from build123d import *

# Parameters (mm, degrees)
F1_DEPTH = 15
F2_R     = 7.63
F3_DEPTH = 15.001


with BuildPart() as f1:
    # F0 (on Front) → F1 (new body)
    with BuildSketch(Plane.XZ):
        Polygon((-7.649891, 13.25), (-15.299782, 0), (-7.649891, -13.25), (7.649891, -13.25), (15.299782, 0), (7.649891, 13.25), align=None)
    extrude(amount=F1_DEPTH)

    # F2 (on face) → F3 (cut, through all)
    with BuildSketch(Plane.XZ.offset(15)):
        Circle(F2_R)
    extrude(amount=-F3_DEPTH, mode=Mode.SUBTRACT)


solid = f1.part
Could you check a few things on this model? Use its own coordinates, in mm. Round coordinates to 2 decimals unless told otherwise and drop trailing zeros. Write each loop counter-clockwise with the first axis right and the second up, starting at its lowest first coordinate (ties: lowest second). Pieces come first, ordered by that corner, then holes. Notation, with made-up numbers: (-25.75, 23) -> (-13.75, 23) arc R5 cw to (-13.75, 30) -> close; hole circle Ø7 at (-13, 48). An arc over 180 degrees is marked (long way). Use a Markdown table: item, result.
1. If we section it at D-D (z = -8.25): List the corners of the cut face in (x, y) for me.
Answer key:
| item | result |
|---|---|
| outline | (-10.54, -15) -> (10.54, -15) -> (10.54, 0) -> (-10.54, 0) -> close |
2. For pin 1 Ø9 at (x, z) = (0, 0) entering from -Y; pin 2 Ø4 at (y, z) = (-3, -10) entering from -X, each with a flat end and sliding along its axis, tell me the tip position at first contact or that it passes through.
Answer key:
| item | result |
|---|---|
| pin 1 | passes through |
| pin 2 | stops at x = -10.68 |
3. If we section it at B-B (y = -9.25): List the corners of the cut face in (x, z) for me, then the cut area to 3 significant figures.
Answer key:
| item | result |
|---|---|
| outline | (-15.3, 0) -> (-7.65, -13.25) -> (7.65, -13.25) -> (15.3, 0) -> (7.65, 13.25) -> (-7.65, 13.25) -> close; hole circle Ø15.26 at (0, 0) |
| area | 425 mm^2 |
4. If we section it at C-C (z = 5): List the corners of the cut face in (x, y) for me, then the cut area to 3 significant figures.
Answer key:
| item | result |
|---|---|
| outline | (-12.41, -15) -> (-5.76, -15) -> (-5.76, 0) -> (-12.41, 0) -> close; (5.76, -15) -> (12.41, -15) -> (12.41, 0) -> (5.76, 0) -> close |
| area | 199 mm^2 |
5. We'd pull the mould along X, two halves only. Please class faces 1 (the face through (-11.53, -7.4, -6.53)), 2 (the face through (11.42, -7.4, -6.72)), 3 (the face through (7.28, -7.6, 2.29)), 4 (the face through (0, -7, 13.25)): +X half, -X half, draft (parallel to the pull), parting line (faces both ways), or undercut.
Answer key:
| item | result |
|---|---|
| face 1 | -X half |
| face 2 | +X half |
| face 3 | undercut |
| face 4 | draft |
6. Please list where these lines run through material, in increasing order: probe 1 along Z at (x, y) = (0, -3.75); probe 2 along Z at (x, y) = (3.5, -2.5); probe 3 along X at (y, z) = (-12.75, -1.5).
Answer key:
| item | result |
|---|---|
| probe 1 | z = -13.25 to -7.63, 7.63 to 13.25 |
| probe 2 | z = -13.25 to -6.78, 6.78 to 13.25 |
| probe 3 | x = -14.43 to -7.48, 7.48 to 14.43 |
7. If we section it at A-A (x = 0): List the corners of the cut face in (y, z) for me, then the cut area to 3 significant figures.
Answer key:
| item | result |
|---|---|
| outline | (-15, -13.25) -> (0, -13.25) -> (0, -7.63) -> (-15, -7.63) -> close; (-15, 7.63) -> (0, 7.63) -> (0, 13.25) -> (-15, 13.25) -> close |
| area | 169 mm^2 |
